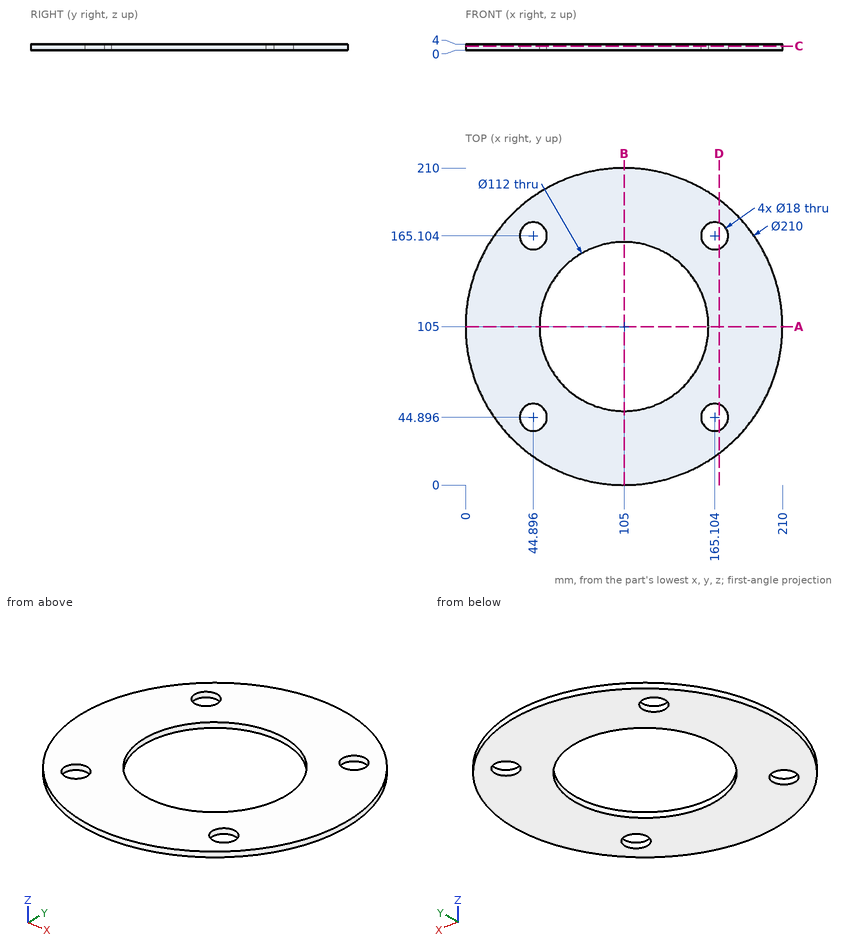
Input: dimensioned drawing with shaded views. Units: mm. Origin: part minimum x, y, z. Coordinates: 2 decimals unless noted, no trailing zeros. Order: outer loops, then holes, each group sorted by start corner. A loop starts at its lowest first (then second) coordinate and runs counter-clockwise, first axis right, second up.
(1) Material intervals for probe 1 along Y at (x, z) = (167, 1); probe 2 along Y at (x, z) = (82.5, 3.55); probe 3 along Y at (x, z) = (38, 1.6) (1 decimal), sorted ascending.
(2) Section query A-A (y = 105). Return the cut outline in (x, z).
(3) First-contact query: pin 1 (1 mm diameter, centred on y = 66, z = 2.5, fed in from +X); pin 2 (14.5 mm diameter, centred on x = 165.1, y = 165.1, fed in from -Z); pin 3 (1 mm diameter, centred on x = 128.5, z = 0.5, fed in from -Y). Flat tips, straight axial feed; report the tip coordinate or a pass-through.
(4) Section query D-D (x = 168). Return the cut outline in (y, z), plus the area to 3 significant figures.
(5) Section query C-C (z = 2.65). Return the cut outline in (x, y).
Solution:
1. probe 1: y = 20.26 to 36.1, 53.69 to 156.31, 173.9 to 189.74
1. probe 2: y = 2.44 to 53.72, 156.28 to 207.56
1. probe 3: y = 24.2 to 39.1, 50.7 to 159.3, 170.9 to 185.8
2. outline: (0, 0) - (49, 0) - (49, 4) - (0, 4) - close; (161, 0) - (210, 0) - (210, 4) - (161, 4) - close
3. pin 1: stops at x = 202.69
3. pin 2: passes through
3. pin 3: stops at y = 2.55
4. outline: (21, 0) - (36.37, 0) - (36.37, 4) - (21, 4) - close; (53.42, 0) - (156.58, 0) - (156.58, 4) - (53.42, 4) - close; (173.63, 0) - (189, 0) - (189, 4) - (173.63, 4) - close
4. area: 536 mm2
5. outline: circle Ø210 at (105, 105); hole circle Ø18 at (44.9, 44.9); hole circle Ø18 at (44.9, 165.1); hole circle Ø112 at (105, 105); hole circle Ø18 at (165.1, 44.9); hole circle Ø18 at (165.1, 165.1)
